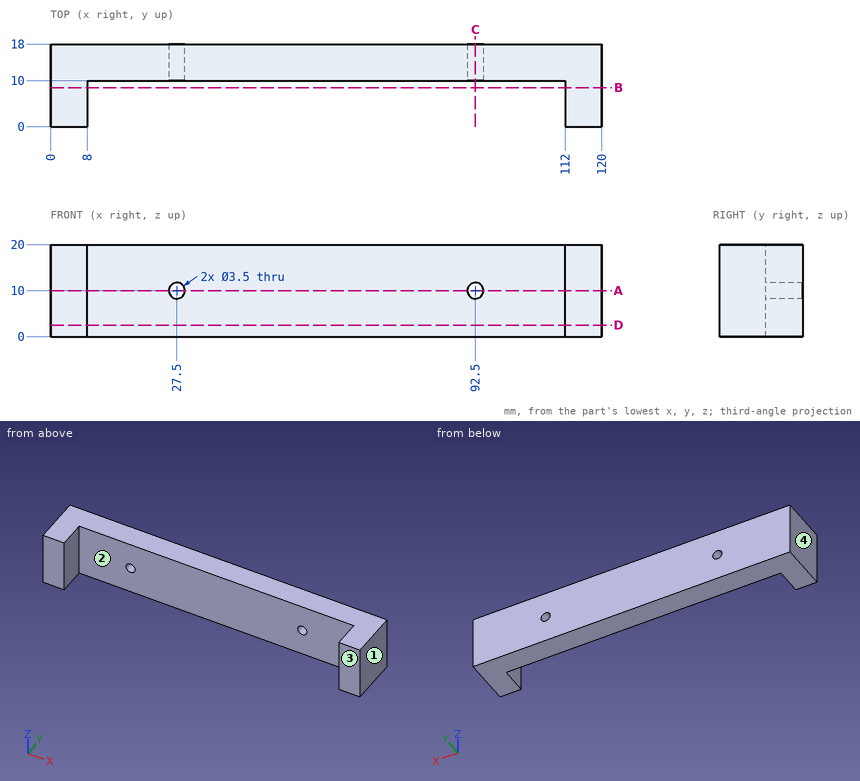
Geometry check sheet. Reference: drawing and pictorial views, mm from the part's lowest x, y, z. Round coordinates to 2 decimals unless told otherwise and drop trailing zeros. Loops run counter-clockwise (first coordinate to the right, second up) from the corner with the lowest first, then second, coordinate; pieces in that order, holes last. Notation, with made-up numbers: M -2.75,19.5 L 5.25,19.5 A22 ccw 5.25,47.5 Z; hole C 40,36 d2. An arc over 180 degrees is marked long. One line per item, written item: value.
(1) Sectioned sample at B-B, the plane y = 8.5. Record the cut outline in (x, z).
Computed values:
outline: M 0,0 L 8,0 L 8,20 L 0,20 Z; M 112,0 L 120,0 L 120,20 L 112,20 Z
(2) Sectioned sample at A-A, the plane z = 10. Record the cut outline in (x, y), then the cut area to 3 significant figures.
Computed values:
outline: M 0,0 L 8,0 L 8,10 L 25.75,10 L 25.75,18 L 0,18 Z; M 29.25,10 L 90.75,10 L 90.75,18 L 29.25,18 Z; M 94.25,10 L 112,10 L 112,0 L 120,0 L 120,18 L 94.25,18 Z
area: 1,060 mm^2
(3) Thickness scan on line 1 (Z direction, x = 92.5, y = 15.25); line 2 (X direction, y = 2.25, z = 7); line 3 (Y direction, x = 108.5, z = 2.75). Record the ranges inside material, lowest first.
Computed values:
line 1: z = 0 to 8.25, 11.75 to 20
line 2: x = 0 to 8, 112 to 120
line 3: y = 10 to 18
(4) Release check for a two-part mould opening along X. For the marked faces 1, 2, 3 and 4 record: +X half, -X half, draft (parallel to the pull), parting line (faces both ways), or undercut.
Computed values:
face 1: +X half
face 2: undercut
face 3: draft
face 4: -X half
(5) Sectioned sample at C-C, the plane x = 92.5. Record the cut outline in (y, z).
Computed values:
outline: M 10,0 L 18,0 L 18,8.25 L 10,8.25 Z; M 10,11.75 L 18,11.75 L 18,20 L 10,20 Z
(6) Depth check by flat-ended pin: pin 1 Ø5 at (x, z) = (54, 16.5) entering from -Y; pin 2 Ø1.5 at (x, y) = (38, 8) entering from -Z. Enter the tip coordinate at first touch or a pass-through.
Computed values:
pin 1: stops at y = 10
pin 2: passes through
(7) Sectioned sample at D-D, the plane z = 2.5. Record the cut outline in (x, y), then the cut area to 3 significant figures.
Computed values:
outline: M 0,0 L 8,0 L 8,10 L 112,10 L 112,0 L 120,0 L 120,18 L 0,18 Z
area: 1,120 mm^2
